```python
from build123d import *


with BuildPart() as part:
    # Sketch1 → Boss-Revolve1 (revolve)
    with BuildSketch(Plane(origin=(0, 0, 0), x_dir=(0, 0, -1), z_dir=(1, 0, 0))):
        Polygon((-1.27, 1.778), (-1.27, -1.1938), (-2.38125, -1.1938), (-2.38125, 0), (-3.556, 0), (-3.556, 1.27), (-3.048, 1.778), align=None)
    revolve(axis=Axis((0, 40, 0), (0, -1, 0)))


solid = part.part
```
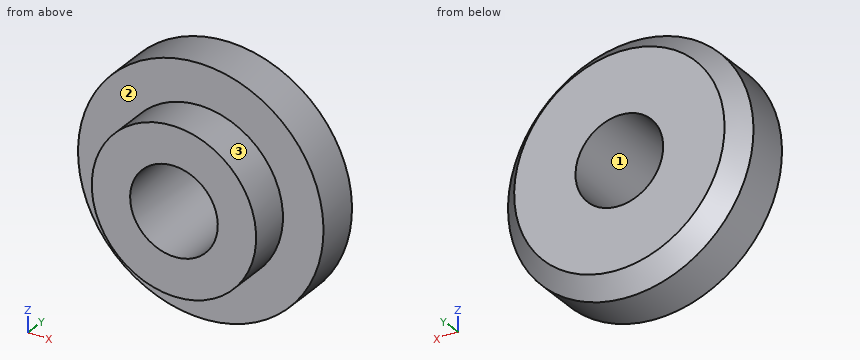
Design review of the part built by this model. Coordinates are the model's own, in mm. Face numbers are marked on the shaded views. Coordinates: 2 decimals unless noted, no trailing zeros. Loops run counter-clockwise (first coordinate to the right, second up) from the corner with the lowest first, then second, coordinate; pieces in that order, holes last. Notation, with made-up numbers: (16.5, -20.5) -> (28.5, -20.5) arc R20 ccw to (28.5, 0.5) -> close; hole circle Ø3 at (80, 35). An arc over 180 degrees is marked (long way). Answer as a JSON object with one key per item and string values.
Q1. The part is to be moulded in two halves that separate along Z. For the marked faces 1, 2 and 3, say which applies: +Z half, -Z half, draft (parallel to the pull), parting line (faces both ways), or undercut.
Answer block:
{"face 1": "undercut", "face 2": "draft", "face 3": "parting line"}
Q2. Take a section at A-A on z = 0. Give the boundary of the cut face in (x, y).
Answer block:
{"outline": "(-3.56, 0) -> (-2.38, 0) -> (-2.38, -1.19) -> (-1.27, -1.19) -> (-1.27, 1.78) -> (-3.05, 1.78) -> (-3.56, 1.27) -> close; (1.27, -1.19) -> (2.38, -1.19) -> (2.38, 0) -> (3.56, 0) -> (3.56, 1.27) -> (3.05, 1.78) -> (1.27, 1.78) -> close"}
Q3. To check wall thickness, follow L1, parallel to Z at x = 0, y = 1; L2, parallel to X at y = -0.2, z = 0. State the ranges of each line that lie inside material, in increasing order.
Answer block:
{"L1": "z = -3.56 to -1.27, 1.27 to 3.56", "L2": "x = -2.38 to -1.27, 1.27 to 2.38"}
Q4. Take a section at B-B on y = 0.15. Give the boundary of the cut face in (x, z), plus the area to 3 significant figures.
Answer block:
{"outline": "circle Ø7.11 at (0, 0); hole circle Ø2.54 at (0, 0)", "area": "34.7 mm^2"}
Q5. Clearance check with flat-ended pins moving along their axes: pin 1 Ø1.5 at (x, z) = (0, 0) entering from +Y; pin 2 Ø1 at (x, y) = (-2, 0.5) entering from +Z. State where each tip first meets the part, or that it passes through.
Answer block:
{"pin 1": "passes through", "pin 2": "stops at z = 3.22"}
